from build123d import *

# Parameters (mm, degrees)
F0_R     = 14.2875
F1_DEPTH = 21.082


with BuildPart() as f1:
    # F0 (on Front) → F1 (new body)
    with BuildSketch(Plane.XZ):
        with BuildLine():
            ThreePointArc((5.042647, -28.126541), (21.916025, -18.336262), (28.575, 0))
            ThreePointArc((28.575, 0), (21.916025, 18.336262), (5.042647, 28.126541))
            ThreePointArc((5.042647, 28.126541), (-28.575, 0), (5.042647, -28.126541))
        make_face()
        with BuildLine():
            ThreePointArc((-13.470384, 4.7625), (0, 14.2875), (13.470384, 4.7625))
            Line((13.470384, 4.7625), (19.05, 4.7625))
            Line((19.05, 4.7625), (19.05, -4.7625))
            Line((19.05, -4.7625), (13.470384, -4.7625))
            ThreePointArc((13.470384, -4.7625), (0, -14.2875), (-13.470384, -4.7625))
            Line((-13.470384, -4.7625), (-19.05, -4.7625))
            Line((-19.05, -4.7625), (-19.05, 4.7625))
            Line((-19.05, 4.7625), (-13.470384, 4.7625))
        make_face(mode=Mode.SUBTRACT)
        with BuildLine():
            ThreePointArc((5.042647, 28.126541), (21.916025, 18.336262), (28.575, 0))
            ThreePointArc((28.575, 0), (21.916025, -18.336262), (5.042647, -28.126541))
            Line((5.042647, -28.126541), (57.336765, -18.751028))
            ThreePointArc((57.336765, -18.751028), (34.925, 0), (57.336765, 18.751028))
            Line((57.336765, 18.751028), (5.042647, 28.126541))
        make_face()
        with BuildLine():
            ThreePointArc((73.025, 0), (68.585683, 12.224174), (57.336765, 18.751028))
            ThreePointArc((57.336765, 18.751028), (34.925, 0), (57.336765, -18.751028))
            ThreePointArc((57.336765, -18.751028), (68.585683, -12.224174), (73.025, 0))
        make_face()
        with Locations((53.975, 0)):
            Circle(F0_R, mode=Mode.SUBTRACT)
        with BuildLine():
            ThreePointArc((-13.470384, -4.7625), (-14.2875, 0), (-13.470384, 4.7625))
            Line((-13.470384, 4.7625), (-19.05, 4.7625))
            Line((-19.05, 4.7625), (-19.05, -4.7625))
            Line((-19.05, -4.7625), (-13.470384, -4.7625))
        make_face()
    extrude(amount=F1_DEPTH)


solid = f1.part
Part model, mm, in its own coordinate system. A direction names the side the tool comes from. Coordinates: 2 decimals unless noted, no trailing zeros. Write each loop counter-clockwise with the first axis right and the second up, starting at its lowest first coordinate (ties: lowest second). Pieces come first, ordered by that corner, then holes. Notation, with made-up numbers: M 19,89.25 L 46,89.25 A20 cw 46,114.25 Z; hole C 72,66 d3. An arc over 180 degrees is marked long. Return JSON: item names as keys, results as strings.
1. Saw through at D-D, the plane z = 22. Write the cut outline in (x, y).
Determined:
{"outline": "M -18.24,-21.08 L 39.21,-21.08 L 39.21,0 L -18.24,0 Z"}
2. 3-axis set-ups, long thin cutter, end or side, ignore diameter. For faces 4 (the face through (22, -21.082, 0)), 5 (the face through (16, -10, 4.762)): which of +Z, -Z, +X, -X, +Y, -Y reach the whole face in a straight line?
Determined:
{"face 4": "+Z, -Z, +X, -X, -Y", "face 5": "+Y, -Y"}
3. Saw through at B-B, the plane z = 12. Write the cut outline in (x, y), then the cut area to 3 significant figures.
Determined:
{"outline": "M -25.93,-21.08 L -7.75,-21.08 L -7.75,0 L -25.93,0 Z; M 7.75,-21.08 L 46.22,-21.08 L 46.22,0 L 7.75,0 Z; M 61.73,-21.08 L 68.77,-21.08 L 68.77,0 L 61.73,0 Z", "area": "1,340 mm²"}
4. Saw through at A-A, the plane x = 0. Write the cut outline in (y, z) (1 decimal).
Determined:
{"outline": "M -21.1,-28.6 L 0,-28.6 L 0,-14.3 L -21.1,-14.3 Z; M -21.1,14.3 L 0,14.3 L 0,28.6 L -21.1,28.6 Z"}
5. Probe L1, parallel to X at y = -16.5, z = 1.5; L2, parallel to X at y = -18, z = -6.5; L3, parallel to Z at x = 49.5, y = -15. List the from-to ranges inside material, lowest first.
Determined:
{"L1": "-28.54 to -14.21, 19.05 to 39.77, 68.18 to 72.97", "L2": "-27.83 to -12.72, 12.72 to 41.25, 66.7 to 71.88", "L3": "-20.16 to -13.57, 13.57 to 20.16"}
6. Pull direction Z, two halves, no side cores. Call faces 1 (the face through (-28.566, -10.393, 0.699)), 2 (the face through (19.05, -10, 0)), 3 (the face through (30.824, -10.393, -23.504)): pulls with the +Z half, pulls with the -Z half, needs draft (parallel to the pull), parting line crosses it, or undercut.
Determined:
{"face 1": "parting line crosses it", "face 2": "undercut", "face 3": "pulls with the -Z half"}
7. Flat gauge pins, fed straight in: pin 1 Ø4 at (y, z) = (-8.5, 23) entering from -X; pin 2 Ø6 at (x, y) = (32, -2.5) entering from -Z; pin 3 Ø5 at (x, y) = (-5.5, -11) entering from -Z. Where does each tip first touch, or does it go through?
Determined:
{"pin 1": "x = -19.38", "pin 2": "z = -23.83", "pin 3": "z = -28.42"}
8. Saw through at C-C, the plane y = -5.25. Count the separate pieces of the cut face and the enclosed holes in it, then the cut area to 3 significant figures.
Determined:
{"separate pieces": "1", "enclosed holes": "2", "area": "3,130 mm²"}
